```python
from build123d import *

# Parameters (mm, degrees)
SKETCH1_R           = 23.5
SKETCH1_R_2         = 21.5
BOSS_EXTRUDE1_DEPTH = 1.5
CUT_EXTRUDE1_REACH  = 25.5


with BuildPart() as part:
    # Sketch1 → Boss-Extrude1 (new body, symmetric)
    with BuildSketch(Plane(origin=(0, 0, 0), x_dir=(1, 0, 0), z_dir=(0, 1, 0))):
        Circle(SKETCH1_R)
        Circle(SKETCH1_R_2, mode=Mode.SUBTRACT)
    extrude(amount=BOSS_EXTRUDE1_DEPTH, both=True)

    # Sketch2 → Cut-Extrude1 (cut, up to next)
    with BuildSketch(Plane(origin=(0, 0, 0), x_dir=(0, 0, -1), z_dir=(1, 0, 0)), mode=Mode.PRIVATE) as cut_extrude1_sk1:
        Polygon((-1.593721188, 1.5), (1.406278812, -1.5), (2.406278812, -1.5), (-0.593721188, 1.5), align=None)
    cut_extrude1_tool1 = extrude(cut_extrude1_sk1.sketch, amount=-CUT_EXTRUDE1_REACH, mode=Mode.PRIVATE) & part.part
    add(cut_extrude1_tool1.solids().sort_by_distance((0, 0, -0.406279))[0], mode=Mode.SUBTRACT)


solid = part.part
```
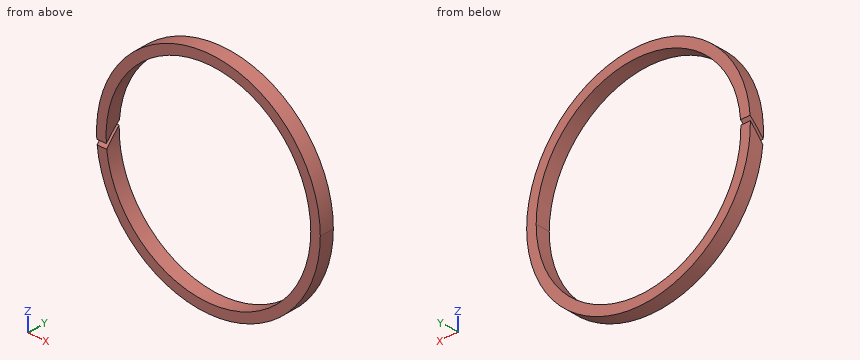
For this review, take the finished solid that the model builds, in its own axes (mm). Round coordinates to 2 decimals unless told otherwise and drop trailing zeros. Write each loop counter-clockwise with the first axis right and the second up, starting at its lowest first coordinate (ties: lowest second). Pieces come first, ordered by that corner, then holes. Notation, with made-up numbers: (34, 56.25) - (84, 56.25) arc R31 cw to (84, 80.25) - close; hole circle Ø8 at (-14.75, 88.5). An arc over 180 degrees is marked (long way). Answer as a JSON object with one key per item and string values.
1. We need section A-A on x = 0. Give the boundary of the cut face in (y, z).
Response values:
{"outline": "(-1.5, -23.5) - (1.5, -23.5) - (1.5, -21.5) - (-1.5, -21.5) - close; (-1.5, 21.5) - (1.5, 21.5) - (1.5, 23.5) - (-1.5, 23.5) - close"}
2. We need section C-C on z = 0. Give the boundary of the cut face in (x, y), then the cut area to 3 significant figures.
Response values:
{"outline": "(-23.5, -1.5) - (-21.5, -1.5) - (-21.5, -0.09) - (-23.5, -0.09) - close; (-23.5, 0.91) - (-21.5, 0.91) - (-21.5, 1.5) - (-23.5, 1.5) - close; (21.5, -1.5) - (23.5, -1.5) - (23.5, 1.5) - (21.5, 1.5) - close", "area": "10.0 mm2"}
3. We need section D-D on y = -0.75. Give the boundary of the cut face in (x, z), then the cut area to 3 significant figures.
Response values:
{"outline": "(-23.49, -0.66) - (-21.49, -0.66) arc R21.5 cw (long way) to (-21.44, -1.66) - (-23.44, -1.66) arc R23.5 ccw (long way) to start", "area": "281 mm2"}
4. For pin 1 Ø1.5 at (y, z) = (0, -2.5) entering from +X; pin 2 Ø8 at (x, z) = (9.5, 10) entering from +Y; pin 3 Ø1 at (y, z) = (0, 17) entering from -X, all flat-tipped, find the tip position at first contact; note any pin that passes through.
Response values:
{"pin 1": "stops at x = 23.43", "pin 2": "passes through", "pin 3": "stops at x = -16.73"}
5. To check wall thickness, follow line 1 along X through (y, z) = (-1.1, 0); line 2 along X through (y, z) = (0.4, 9.5); line 3 along Z through (x, y) = (1, -0.6). State the ranges of each line that lie inside material, in increasing order.
Response values:
{"line 1": "x = -23.5 to -21.5, 21.5 to 23.5", "line 2": "x = -21.49 to -19.29, 19.29 to 21.49", "line 3": "z = -23.48 to -21.48, 21.48 to 23.48"}
6. We need section B-B on z = 5. Give the boundary of the cut face in (x, y).
Response values:
{"outline": "(-22.96, -1.5) - (-20.91, -1.5) - (-20.91, 1.5) - (-22.96, 1.5) - close; (20.91, -1.5) - (22.96, -1.5) - (22.96, 1.5) - (20.91, 1.5) - close"}
